Here's how the part is built. I have some questions about the finished solid (model axes, mm). A direction names the side the tool comes from. Coordinates: 2 decimals unless noted, no trailing zeros. Write each loop counter-clockwise with the first axis right and the second up, starting at its lowest first coordinate (ties: lowest second). Pieces come first, ordered by that corner, then holes.
Item 1: We'd pull the mould along Z, two halves only. Please class faces 1 (the face through (-14.579, 43.198, -16.345)), 2 (the face through (20, 23, 19)), 3 (the face through (20, 23, -19)): +Z half, -Z half, draft (parallel to the pull), parting line (faces both ways), or undercut.
Item 2: If we section it at B-B (z = 0): Please give me the cut outline in (x, y), then the cut area to 3 significant figures.
Item 3: If we section it at A-A (x = 0): Please give me the cut outline in (y, z), then the cut area to 3 significant figures.
Item 4: If I drill on line 1 (X direction, y = 41, z = -15.5); line 2 (Z direction, x = -15, y = 43), over which ranges is the centre line in solid material (lowest first)?
Item 5: I'm going to push flat-ended pins straight in: pin 1 Ø1.5 at (x, z) = (1, -5.5) entering from -Y; pin 2 Ø1.5 at (x, z) = (-5.5, 14) entering from +Y; pin 3 Ø3 at (x, z) = (-15.5, -15.5) entering from +Y; pin 4 Ø1.5 at (x, y) = (-2.5, 51.5) entering from +Z. Where does each tip first touch, or does it pass through?
Item 6: For faces 4 (the face through (0, 23, 21)), 5 (the face through (-2.44, 59.35, -0.54)), which set-ups out of +Z, -Z, +X, -X, +Y, -Y let a thin tool reach every point of the face, with its end or its side?
Item 7: If we section it at C-C (y = 53.5): Please give me the cut outline in (x, z).
Item 8: If we section it at D-D (x = 10): Please give me the cut outline in (y, z).
from build123d import *

# Parameters (mm, degrees)
SKETCH_1_W             = 42
SKETCH_1_H             = 42
EXTRUDE_1_DEPTH        = 47
SKETCH_2_R             = 16.25
CUT_EXTRUDE_1_DEPTH    = 0.5
SKETCH_3_R             = 11
EXTRUDE_2_DEPTH        = 2
SKETCH_4_R             = 2.5
EXTRUDE_3_DEPTH        = 22
CHAMFER_1_SIZE         = 3
HOLE_WIZARD_M3_1_D     = 2.5
HOLE_WIZARD_M3_1_DEPTH = 7.5
HOLE_WIZARD_M3_1_TIP   = 0.751075774


with BuildPart() as part:
    # 草圖1 → 填料-伸長1 (new body)
    with BuildSketch(Plane(origin=(0, 0, 0), x_dir=(1, 0, 0), z_dir=(0, 1, 0))):
        Rectangle(SKETCH_1_W, SKETCH_1_H)
    extrude(amount=EXTRUDE_1_DEPTH)

    # 草圖2 → 除料-伸長1 (cut)
    with BuildSketch(Plane(origin=(0, 47, 0), x_dir=(1, 0, 0), z_dir=(0, 1, 0))):
        with Locations(Location((0, 0, 0), (0, 0, 270))):
            Circle(SKETCH_2_R)
    extrude(amount=-CUT_EXTRUDE_1_DEPTH, mode=Mode.SUBTRACT)

    # 草圖3 → 填料-伸長2 (add)
    with BuildSketch(Plane(origin=(0, 46.5, 0), x_dir=(1, 0, 0), z_dir=(0, 1, 0))):
        with Locations(Location((0, 0, 0), (0, 0, 270))):
            Circle(SKETCH_3_R)
    extrude(amount=EXTRUDE_2_DEPTH)

    # 草圖4 → 填料-伸長3 (add)
    with BuildSketch(Plane(origin=(0, 48.5, 0), x_dir=(1, 0, 0), z_dir=(0, 1, 0))):
        with Locations(Location((0, 0, 0), (0, 0, 270))):
            Circle(SKETCH_4_R)
    extrude(amount=EXTRUDE_3_DEPTH)

    # 導角1
    chamfer_1_edges = [part.edges().sort_by_distance(p)[0] for p in [
        (21, 23.5, 21),
        (-21, 23.5, 21),
        (-21, 23.5, -21),
        (21, 23.5, -21),
    ]]
    chamfer(chamfer_1_edges, length=CHAMFER_1_SIZE)

    # M3 螺紋孔1
    with Locations(Plane(origin=(0, 47, 0), x_dir=(1, 0, 0), z_dir=(0, 1, 0))):
        with Locations((-15.5, 15.5), (-15.5, -15.5), (15.5, 15.5), (15.5, -15.5)):
            Hole(HOLE_WIZARD_M3_1_D / 2, depth=HOLE_WIZARD_M3_1_DEPTH)
            with Locations((0, 0, -(HOLE_WIZARD_M3_1_DEPTH + HOLE_WIZARD_M3_1_TIP / 2))):  # 118° drill point
                Cone(0, HOLE_WIZARD_M3_1_D / 2, HOLE_WIZARD_M3_1_TIP, mode=Mode.SUBTRACT)


solid = part.part
Answer list:
1. face 1: undercut
1. face 2: +Z half
1. face 3: -Z half
2. outline: (-21, 0) - (21, 0) - (21, 47) - (16.25, 47) - (16.25, 46.5) - (11, 46.5) - (11, 48.5) - (2.5, 48.5) - (2.5, 70.5) - (-2.5, 70.5) - (-2.5, 48.5) - (-11, 48.5) - (-11, 46.5) - (-16.25, 46.5) - (-16.25, 47) - (-21, 47) - close
2. area: 2,110 mm2
3. outline: (0, -21) - (47, -21) - (47, -16.25) - (46.5, -16.25) - (46.5, -11) - (48.5, -11) - (48.5, -2.5) - (70.5, -2.5) - (70.5, 2.5) - (48.5, 2.5) - (48.5, 11) - (46.5, 11) - (46.5, 16.25) - (47, 16.25) - (47, 21) - (0, 21) - close
3. area: 2,110 mm2
4. line 1: x = -21 to -16.75, -14.25 to 14.25, 16.75 to 21
4. line 2: z = -21 to -16.65, -14.35 to 14.35, 16.65 to 21
5. pin 1: stops at y = 0
5. pin 2: stops at y = 46.5
5. pin 3: stops at y = 47
5. pin 4: stops at z = 1.79
6. face 4: +Z, +X, -X, +Y, -Y
6. face 5: +Y
7. outline: circle Ø5 at (0, 0)
8. outline: (0, -21) - (47, -21) - (47, -12.81) - (46.5, -12.81) - (46.5, -4.58) - (48.5, -4.58) - (48.5, 4.58) - (46.5, 4.58) - (46.5, 12.81) - (47, 12.81) - (47, 21) - (0, 21) - close
